Geometry: final body of the model. Coordinates: model frame, mm. A direction names the side the tool comes from. Coordinates: 2 decimals unless noted, no trailing zeros. Write each loop counter-clockwise with the first axis right and the second up, starting at its lowest first coordinate (ties: lowest second). Pieces come first, ordered by that corner, then holes. Notation, with made-up numbers: (-2, 74) -> (4, 74) arc R10 ccw to (4, 89) -> close; hole circle Ø6 at (78, 60.5). An arc over 180 degrees is marked (long way). One line per item, written item: value.
```python
from build123d import *

# Parameters (mm, degrees)
SKETCH001_R        = 1.7
POCKET_DEPTH       = 136.636862
POCKET_DEPTH_BACK  = 136.636862
POCKET001_DEPTH    = 133.636862
POLARPATTERN_COUNT = 4


with BuildPart() as part:
    # Sketch → Revolution (revolve)
    with BuildSketch(Plane.XZ):
        with BuildLine():
            Line((14, -5), (14, -3))
            ThreePointArc((14, -3), (13.707107, -2.292893), (13, -2))
            Line((13, -2), (2.7, -2))
            Line((2.7, -2), (2.7, 5))
            Line((2.7, 5), (21, 5))
            ThreePointArc((21, -5), (23, 0), (21, 5))
            Line((21, -5), (14, -5))
        make_face()
    revolve(axis=Axis((0, 0, 0), (0, 0, 1)))

    # Sketch001 → Pocket (cut, two sides)
    with BuildSketch(Plane(origin=(0, 9.5, 0), x_dir=(1, 0, 0), z_dir=(0, 0, 1))) as pocket_sk:
        Circle(SKETCH001_R)
    pocket = extrude(amount=-POCKET_DEPTH, mode=Mode.SUBTRACT) + extrude(pocket_sk.sketch, amount=POCKET_DEPTH_BACK, mode=Mode.SUBTRACT)

    # Sketch002 (on Sketch) → Pocket001 (cut, through all)
    with BuildSketch(Plane(origin=(0, 9.5, 3), x_dir=(1, 0, 0), z_dir=(0, 0, 1))):
        Polygon((1.732051, -3), (3.464102, 0), (1.732051, 3), (-1.732051, 3), (-3.464102, 0), (-1.732051, -3), align=None)
    pocket001 = extrude(amount=POCKET001_DEPTH, mode=Mode.SUBTRACT)

    # PolarPattern: Pocket, Pocket001 ×4 about axis
    polarpattern_axis = Axis((0, 0, 0), (0, 0, 1))
    for i in range(1, POLARPATTERN_COUNT):
        add(pocket.rotate(polarpattern_axis, i * 360 / POLARPATTERN_COUNT), mode=Mode.SUBTRACT)
        add(pocket001.rotate(polarpattern_axis, i * 360 / POLARPATTERN_COUNT), mode=Mode.SUBTRACT)


solid = part.part
```
(1) Section A-A (y = 0). State how many separate pieces and enclosed holes the cut face has, then the cut area to 3 significant figures.
Responses:
separate pieces: 4
enclosed holes: 0
area: 268 mm2
(2) Pull-direction query (X, two-part tool) for faces 4 (the flat face through (4, -14, -5)), 5 (the flat face through (2.6, -8, 4)); classes: released by +X, released by -X, zero draft, split by the parting line, or undercut.
Responses:
face 4: zero draft
face 5: undercut
(3) Reachability of faces 1 (the cylindrical face through (12.932, -5.362, -3.986)), 2 (the flat face through (2.6, 8, 4)), 3 (the cylindrical face through (-0.37, 7.84, 0.54)) from +Z, -Z, +X, -X, +Y, -Y: full face, straight path, thin tool, end or side. Return the list, or none.
Responses:
face 1: -Z
face 2: +Z
face 3: +Z, -Z
(4) First-contact query: pin 1 (2 mm diameter, centred on y = 0.5, z = 4.5, fed in from -X); pin 2 (4 mm diameter, centred on y = 13, z = 1, fed in from -X); pin 3 (2 mm diameter, centred on x = 0, y = -9.5, fed in from +Z); pin 4 (2 mm diameter, centred on x = 1, z = 4.5, fed in from +Y). Flat tips, straight axial feed; report the tip coordinate or a pass-through.
Responses:
pin 1: stops at x = -22.09
pin 2: stops at x = -20.15
pin 3: passes through
pin 4: stops at y = 22.08
(5) Line query: line 1 (Y direction, x = 0, z = 0.6); line 2 (Y direction, x = 0, z = 1.5); line 3 (Z direction, x = -5, y = 2). Output: solid intervals per line, ascending. Write a range as [from, to].
Responses:
line 1: y = [-22.98, -11.2], [-7.8, -2.7], [2.7, 7.8], [11.2, 22.98]
line 2: y = [-22.84, -11.2], [-7.8, -2.7], [2.7, 7.8], [11.2, 22.84]
line 3: z = [-2, 5]
(6) Section C-C (z = 1.5). Return the cut outline in (x, y), then the cut area to 3 significant figures.
Responses:
outline: circle Ø45.69 at (0, 0); hole circle Ø3.4 at (-9.5, 0); hole circle Ø5.4 at (0, 0); hole circle Ø3.4 at (0, -9.5); hole circle Ø3.4 at (0, 9.5); hole circle Ø3.4 at (9.5, 0)
area: 1,580 mm2
